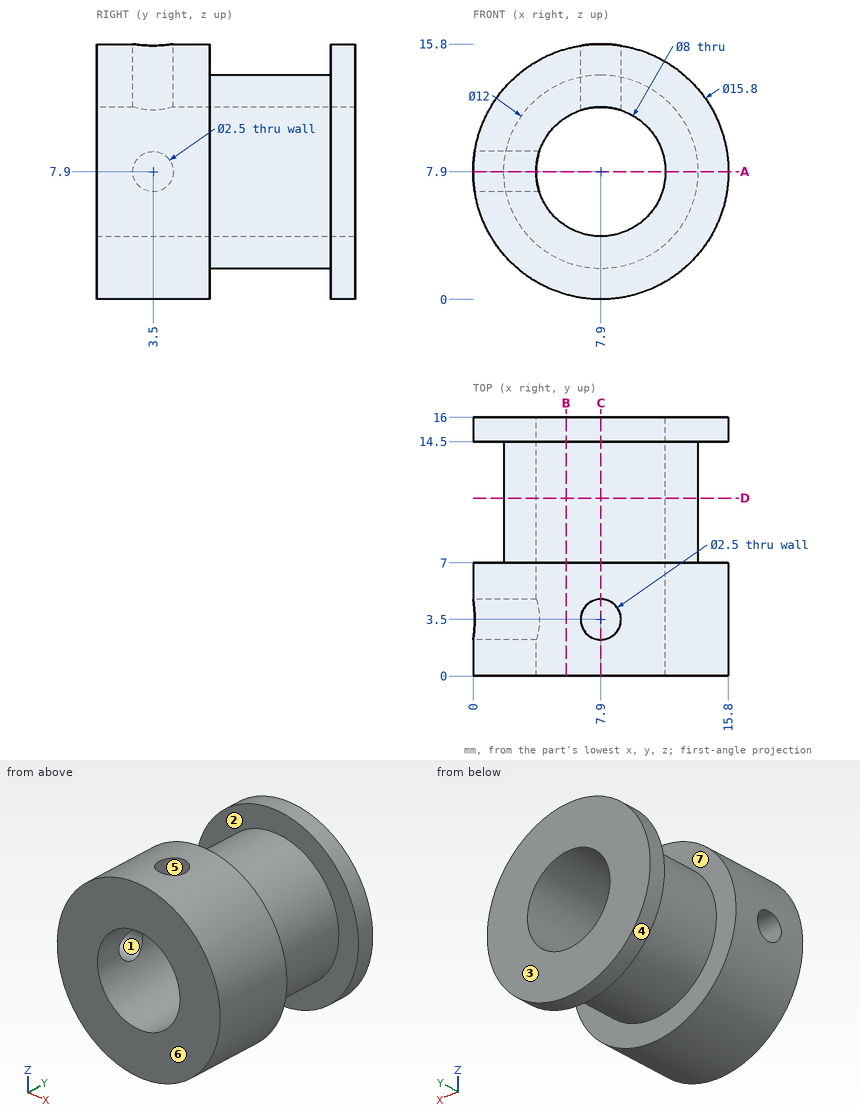
The figure shows three views and two pictorial views of one solid part (mm, origin at its lowest corner). Answer the questions. A direction names the side the tool comes from. Round coordinates to 2 decimals unless told otherwise and drop trailing zeros. Write each loop counter-clockwise with the first axis right and the second up, starting at its lowest first coordinate (ties: lowest second). Pieces come first, ordered by that corner, then holes. Notation, with made-up numbers: M 0.5,-14 L 30.5,-14 A29 cw 30.5,14 Z; hole C 54,36.5 d5. An arc over 180 degrees is marked long. Use a Markdown table: item, result.
1) Determine the mould class of the marked faces 1, 2, 3 and 4 for opening direction Y: pulls with the +Y half, pulls with the -Y half, needs draft (parallel to the pull), parting line crosses it, or undercut.
Taken from the geometry:
| item | result |
|---|---|
| face 1 | undercut |
| face 2 | undercut |
| face 3 | pulls with the +Y half |
| face 4 | needs draft |
2) The part is cut by section B-B on x = 5.75. Give the vertices of the cut face in (y, z), plus the area to 3 significant figures.
Taken from the geometry:
| item | result |
|---|---|
| outline | M 0,0.3 L 7,0.3 L 7,2.3 L 14.5,2.3 L 14.5,0.3 L 16,0.3 L 16,4.53 L 0,4.53 Z; M 0,11.27 L 16,11.27 L 16,15.5 L 14.5,15.5 L 14.5,13.5 L 7,13.5 L 7,15.5 L 0,15.5 Z |
| area | 105 mm2 |
3) The part is cut by section A-A on z = 7.9. Give the vertices of the cut face in (x, y), plus the area to 4 significant figures.
Taken from the geometry:
| item | result |
|---|---|
| outline | M 0,0 L 3.9,0 L 3.9,2.25 L 0,2.25 Z; M 0,4.75 L 3.9,4.75 L 3.9,16 L 0,16 L 0,14.5 L 1.9,14.5 L 1.9,7 L 0,7 Z; M 11.9,0 L 15.8,0 L 15.8,7 L 13.9,7 L 13.9,14.5 L 15.8,14.5 L 15.8,16 L 11.9,16 Z |
| area | 86.55 mm2 |
4) Consider line 1 (X direction, y = 7.75, z = 7.9); line 2 (X direction, y = 5.5, z = 7.9); line 3 (Y direction, x = 12, z = 14.5). Determine where each line is inside the solid, lowest interval first. Write a range as [from, to].
Taken from the geometry:
| item | result |
|---|---|
| line 1 | x = [1.9, 3.9], [11.9, 13.9] |
| line 2 | x = [0, 3.9], [11.9, 15.8] |
| line 3 | y = [0, 7], [14.5, 16] |
5) Which of the six approach directions +Z, -Z, +X, -X, +Y, -Y give full straight-line access (tool end or side, diameter ignored) to the marked faces 5, 6 and 7?
Taken from the geometry:
| item | result |
|---|---|
| face 5 | +Z |
| face 6 | +Z, -Z, +X, -X, -Y |
| face 7 | none |
6) Flat-ended cylindrical pins translate along their axes: pin 1 (1.5 mm diameter, centred on x = 11, y = 4.5, fed in from +Z); pin 2 (1.5 mm diameter, centred on y = 4, z = 9.5, fed in from -X). Find the tip coordinate at first contact, or state that the pin passes through.
Taken from the geometry:
| item | result |
|---|---|
| pin 1 | stops at z = 15.44 |
| pin 2 | stops at x = 0.05 |
7) The part is cut by section D-D on y = 11. Give the vertices of the cut face in (x, z), plus the area to 3 significant figures.
Taken from the geometry:
| item | result |
|---|---|
| outline | C 7.9,7.9 d12; hole C 7.9,7.9 d8 |
| area | 62.8 mm2 |
8) The part is cut by section C-C on x = 7.9. Give the vertices of the cut face in (y, z), plus the area to 4 significant figures.
Taken from the geometry:
| item | result |
|---|---|
| outline | M 0,0 L 7,0 L 7,1.9 L 14.5,1.9 L 14.5,0 L 16,0 L 16,3.9 L 0,3.9 Z; M 0,11.9 L 2.25,11.9 L 2.25,15.8 L 0,15.8 Z; M 4.75,11.9 L 16,11.9 L 16,15.8 L 14.5,15.8 L 14.5,13.9 L 7,13.9 L 7,15.8 L 4.75,15.8 Z |
| area | 86.55 mm2 |
